Answer from the drawing. Dimensions are ordinates in mm from the lowest x, y and z of the part. Coordinates: 2 decimals unless noted, no trailing zeros. Order: outer loops, then holes, each group sorted by start corner. A loop starts at its lowest first (then second) coordinate and runs counter-clockwise, first axis right, second up. Notation, with made-up numbers: (26, 84.25) -> (63, 84.25) arc R29 cw to (63, 105.25) -> close; hole circle Ø2 at (21.25, 70). An arc over 180 degrees is marked (long way). Answer as a JSON object with one key per item and string values. Group by question number.
1) Given pin 1 (1 mm diameter, centred on y = 1, z = 40, fed in from -X); pin 2 (4 mm diameter, centred on x = 10, z = 60, fed in from +Y); pin 3 (1 mm diameter, centred on y = 1, z = 23, fed in from +X), each flat-ended and moving along its own axis, determine where each tip first touches the part or whether it passes through.
2) Section B-B on y = 1.05 is taken. Determine the outline of the cut face in (x, z).
3) Section C-C on x = 41 is taken. Determine the outline of the cut face in (y, z) (1 decimal).
4) Section A-A on z = 40 is taken. Determine the outline of the cut face in (x, y).
5) Consider L1, parallel to Z at x = 25, y = 0.8; L2, parallel to Z at x = 26, y = 1.05 (1 decimal); L3, parallel to X at y = 2.9, z = 60.5. Determine where each line is inside the solid, lowest interval first.
6) Section D-D on z = 29.5 is taken. Determine the outline of the cut face in (x, y).
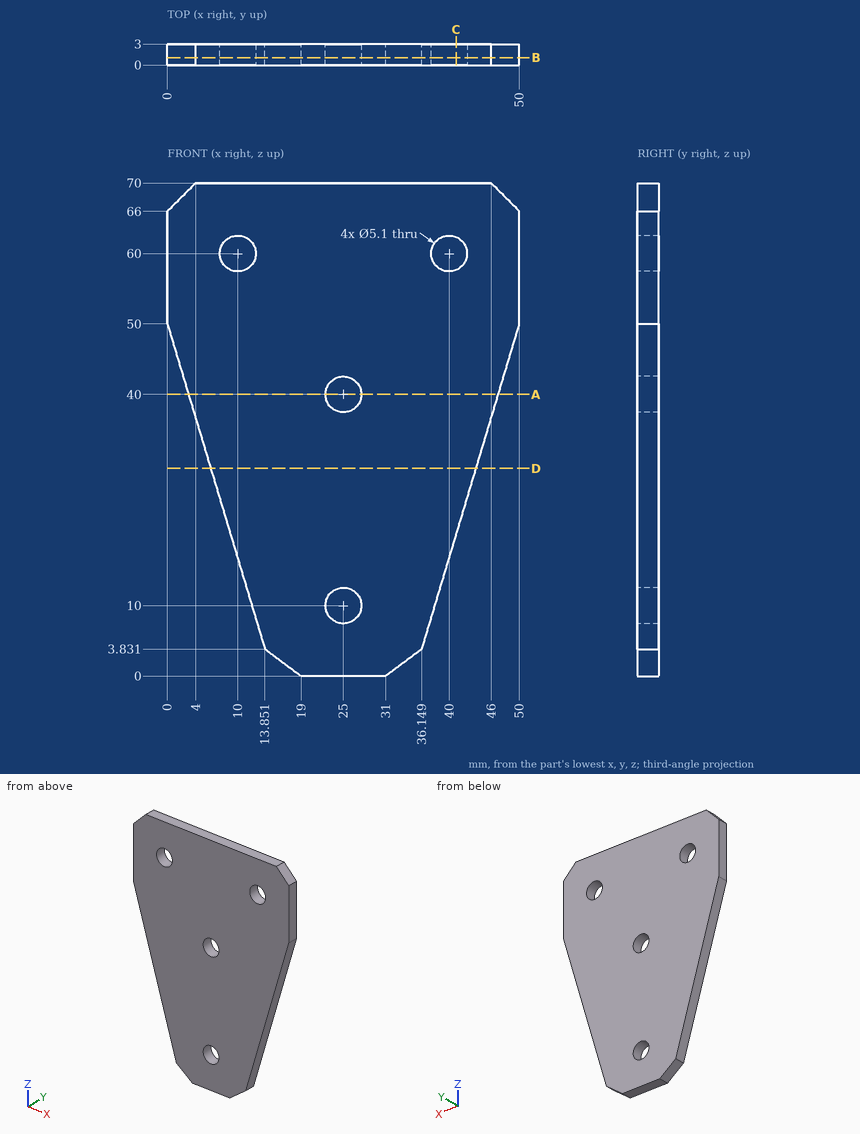
Worked answers:
{
 "1": {"pin 1": "stops at x = 2.85", "pin 2": "passes through", "pin 3": "stops at x = 42.05"},
 "2": {"outline": "(0, 50) -> (13.85, 3.83) -> (19, 0) -> (31, 0) -> (36.15, 3.83) -> (50, 50) -> (50, 66) -> (46, 70) -> (4, 70) -> (0, 66) -> close; hole circle Ø5.1 at (10, 60); hole circle Ø5.1 at (25, 10); hole circle Ø5.1 at (25, 40); hole circle Ø5.1 at (40, 60)"},
 "3": {"outline": "(0, 20) -> (3, 20) -> (3, 57.7) -> (0, 57.7) -> close; (0, 62.3) -> (3, 62.3) -> (3, 70) -> (0, 70) -> close"},
 "4": {"outline": "(3, 0) -> (22.45, 0) -> (22.45, 3) -> (3, 3) -> close; (27.55, 0) -> (47, 0) -> (47, 3) -> (27.55, 3) -> close"},
 "5": {"L1": "z = 0 to 7.45, 12.55 to 37.45, 42.55 to 70", "L2": "z = 0 to 7.7, 12.3 to 37.7, 42.3 to 70", "L3": "x = 0 to 7.5, 12.5 to 37.5, 42.5 to 50"},
 "6": {"outline": "(6.15, 0) -> (43.85, 0) -> (43.85, 3) -> (6.15, 3) -> close"}
}
